from build123d import *

# Parameters (mm, degrees)
SKETCH3_R           = 80
BOSS_EXTRUDE3_DEPTH = 4
SKETCH5_R           = 1.65
CUT_EXTRUDE3_DEPTH  = 114.207773585
CUT_EXTRUDE4_DEPTH  = 114.207773585
CIRPATTERN2_COUNT   = 4
FILLET2_R           = 3
BOSS_EXTRUDE4_START = 15
SKETCH7_R           = 80
SKETCH7_R_2         = 76
BOSS_EXTRUDE4_DEPTH = 15
SKETCH8_R           = 2.2
CUT_EXTRUDE5_DEPTH  = 115.721401665
SKETCH9_R           = 80
SKETCH9_R_2         = 76
BOSS_EXTRUDE5_DEPTH = 15


with BuildPart() as part:
    # Sketch3 → Boss-Extrude3 (new body)
    with BuildSketch(Plane.YZ):
        with Locations(Location((0, 0, 0), (0, 0, 270))):
            Circle(SKETCH3_R)
    extrude(amount=BOSS_EXTRUDE3_DEPTH)

    # Sketch5 → Cut-Extrude3 (cut, through all)
    with BuildSketch(Plane.YZ.offset(4)):
        with Locations(Location((0, 6, 0), (0, 0, 270))):
            Circle(SKETCH5_R)
        with Locations(Location((6, 0, 0), (0, 0, 270))):
            Circle(SKETCH5_R)
        with Locations(Location((0, -6, 0), (0, 0, 270))):
            Circle(SKETCH5_R)
        with Locations(Location((-6, 0, 0), (0, 0, 270))):
            Circle(SKETCH5_R)
    extrude(amount=-CUT_EXTRUDE3_DEPTH, mode=Mode.SUBTRACT)

    # Sketch6 → Cut-Extrude4 (cut, through all)
    with BuildSketch(Plane.YZ.offset(4)):
        with BuildLine():
            Line((11.456439237, 5), (69.821200219, 5))
            ThreePointArc((69.821200219, 5), (49.497474683, 49.497474683), (5, 69.821200219))
            Line((5, 69.821200219), (5, 11.456439237))
            ThreePointArc((5, 11.456439237), (8.838834765, 8.838834765), (11.456439237, 5))
        make_face()
    cut_extrude4 = extrude(amount=-CUT_EXTRUDE4_DEPTH, mode=Mode.SUBTRACT)

    # CirPattern2: Cut-Extrude4 ×4 about axis
    cirpattern2_axis = Axis((0, 0, 0), (1, 0, 0))
    for i in range(1, CIRPATTERN2_COUNT):
        add(cut_extrude4.rotate(cirpattern2_axis, i * 360 / CIRPATTERN2_COUNT), mode=Mode.SUBTRACT)

    # Fillet2
    fillet2_edges = [part.edges().sort_by_distance(p)[0] for p in [
        (2, 5, 69.821200219),
        (2, 69.821200219, 5),
        (2, 69.821200219, -5),
        (2, 5, -69.821200219),
        (2, -5, -69.821200219),
        (2, -69.821200219, -5),
        (2, -69.821200219, 5),
        (2, -5, 69.821200219),
    ]]
    fillet(fillet2_edges, radius=FILLET2_R)

    # Sketch7 → Boss-Extrude4 (add)
    with BuildSketch(Plane(origin=(0, 0, 0), x_dir=(0, -1, 0), z_dir=(-1, 0, 0)).offset(BOSS_EXTRUDE4_START)):
        with Locations(Location((0, 0, 0), (0, 0, 90))):
            Circle(SKETCH7_R)
        with Locations(Location((0, 0, 0), (0, 0, 90))):
            Circle(SKETCH7_R_2, mode=Mode.SUBTRACT)
    extrude(amount=-BOSS_EXTRUDE4_DEPTH)

    # Sketch8 → Cut-Extrude5 (cut, through all)
    with BuildSketch(Plane.YZ.offset(4)):
        with Locations(Location((0, 0, 0), (0, 0, 270))):
            Circle(SKETCH8_R)
    extrude(amount=-CUT_EXTRUDE5_DEPTH, mode=Mode.SUBTRACT)

    # Sketch9 → Boss-Extrude5 (add)
    with BuildSketch(Plane.YZ.offset(4)):
        with Locations(Location((0, 0, 0), (0, 0, 90))):
            Circle(SKETCH9_R)
        with Locations(Location((0, 0, 0), (0, 0, 90))):
            Circle(SKETCH9_R_2, mode=Mode.SUBTRACT)
    extrude(amount=BOSS_EXTRUDE5_DEPTH)


solid = part.part
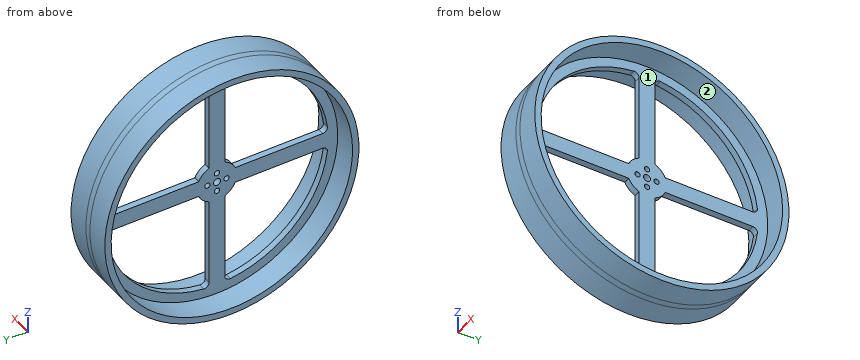
For this review, take the finished solid that the model builds, in its own axes (mm). Face numbers are marked on the shaded views. Round coordinates to 2 decimals unless told otherwise and drop trailing zeros. Order: outer loops, then holes, each group sorted by start corner. A loop starts at its lowest first (then second) coordinate and runs counter-clockwise, first axis right, second up. Notation, with made-up numbers: (17, -9) -> (34, -9) arc R11 cw to (34, 10) -> close; hole circle Ø10 at (80.25, 25.25). An arc over 180 degrees is marked (long way). Put each result on its own line as item: value.
Q1. Mouldability with a two-part tool opening along Y and no side actions: class the marked faces 1 and 2 as pulls with the +Y half, pulls with the -Y half, needs draft (parallel to the pull), parting line crosses it, or undercut.
Check result:
face 1: undercut
face 2: undercut
Q2. Insertion check: pin 1 Ø12 at (x, z) = (-8, -61) entering from -Y; pin 2 Ø2 at (x, z) = (1.5, 32) entering from -Y; pin 3 Ø2 at (x, z) = (1, -43) entering from -Y. Each pin has a flat end and moves straight along its axis. Give the tip position at first contact, or say it passes through.
Check result:
pin 1: y = -58.09
pin 2: y = -73.75
pin 3: y = -68.09
Q3. For probe 1 along Y at (x, z) = (1.4, 0); probe 2 along Y at (x, z) = (-9, 0); probe 3 along X at (y, z) = (53.5, 45.5), list the stretches that pass through material, from the lowest coordinate up. Write a range as [from, to].
Check result:
probe 1: [-80, -7.65], [-4.35, -2.2], [2.2, 4.35], [7.65, 80]
probe 2: [-80, -76], [76, 80]
probe 3: [0, 4]
Q4. Add section A-A on z = 26. Write out the cut boundary in (x, y).
Check result:
outline: (-15, -75.66) -> (19, -75.66) -> (19, -71.41) -> (4, -71.41) -> (4, -64.99) -> (0, -64.99) -> (0, -71.41) -> (-15, -71.41) -> close; (-15, 71.41) -> (0, 71.41) -> (0, 64.99) -> (4, 64.99) -> (4, 71.41) -> (19, 71.41) -> (19, 75.66) -> (-15, 75.66) -> close; (0, -5) -> (4, -5) -> (4, 5) -> (0, 5) -> close
Q5. Add section B-B on y = -33.5. Write out the cut boundary in (x, z), plus the area to 3 significant figures.
Check result:
outline: (-15, -72.65) -> (19, -72.65) -> (19, -68.22) -> (4, -68.22) -> (4, -61.46) -> (0, -61.46) -> (0, -68.22) -> (-15, -68.22) -> close; (-15, 68.22) -> (0, 68.22) -> (0, 61.46) -> (4, 61.46) -> (4, 68.22) -> (19, 68.22) -> (19, 72.65) -> (-15, 72.65) -> close; (0, -5) -> (4, -5) -> (4, 5) -> (0, 5) -> close
area: 395 mm2
Q6. Add section C-C on x = -11.5. Write out the cut boundary in (y, z), plus the area to 3 significant figures.
Check result:
outline: circle Ø160 at (0, 0); hole circle Ø152 at (0, 0)
area: 1,960 mm2
